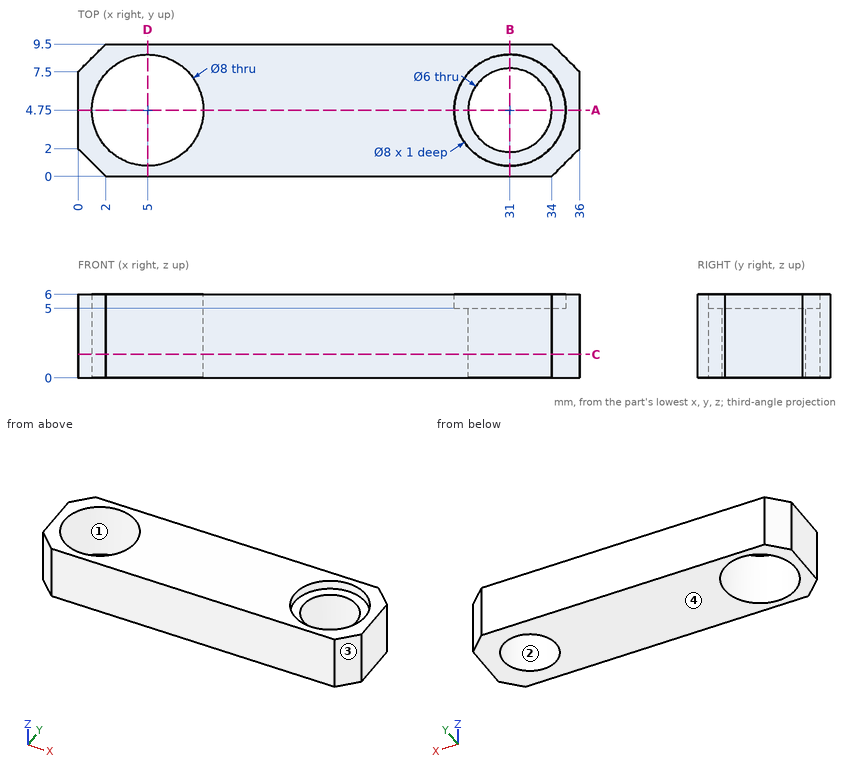
The drawing under review shows one solid part. Ordinate dimensions are in mm from its lowest x, y, z. Round coordinates to 2 decimals unless told otherwise and drop trailing zeros. Loops run counter-clockwise (first coordinate to the right, second up) from the corner with the lowest first, then second, coordinate; pieces in that order, holes last. Notation, with made-up numbers: (16.5, 41.25) - (50.5, 41.25) arc R26 ccw to (50.5, 71.25) - close; hole circle Ø9 at (38.25, 82). An arc over 180 degrees is marked (long way). Use a Markdown table: item, result. Add a question column.
Q1. For probe 1 along X at (y, z) = (4.25, 2.8); probe 2 along X at (y, z) = (7, 3.25); probe 3 along Y at (x, z) = (31, 5.2), list the stretches that pass through material, from the lowest coordinate up.
Q2. Add section C-C (z = 1.7). State the section outline as (x, y) points, plus the area to 3 significant figures.
Q3. The part is to be moulded in two halves that separate along X. For the marked faces 1, 2, 3 and 4, say which applies: pulls with the +X half, pulls with the -X half, needs draft (parallel to the pull), parting line crosses it, or undercut.
Q4. Add section D-D (x = 5). State the section outline as (y, z) points.
Q5. Add section B-B (x = 31). State the section outline as (y, z) points.
Q6. Add section A-A (y = 4.75). State the section outline as (x, z) points.
Worked answers:
| question | item | result |
|---|---|---|
| 1 | probe 1 | 0 to 1.03, 8.97 to 28.04, 33.96 to 36 |
| 1 | probe 2 | 0 to 1.69, 8.31 to 29.02, 32.98 to 36 |
| 1 | probe 3 | 0 to 0.75, 8.75 to 9.5 |
| 2 | outline | (0, 2) - (2, 0) - (34, 0) - (36, 2) - (36, 7.5) - (34, 9.5) - (2, 9.5) - (0, 7.5) - close; hole circle Ø8 at (5, 4.75); hole circle Ø6 at (31, 4.75) |
| 2 | area | 255 mm² |
| 3 | face 1 | undercut |
| 3 | face 2 | undercut |
| 3 | face 3 | pulls with the +X half |
| 3 | face 4 | needs draft |
| 4 | outline | (0, 0) - (0.75, 0) - (0.75, 6) - (0, 6) - close; (8.75, 0) - (9.5, 0) - (9.5, 6) - (8.75, 6) - close |
| 5 | outline | (0, 0) - (1.75, 0) - (1.75, 5) - (0.75, 5) - (0.75, 6) - (0, 6) - close; (7.75, 0) - (9.5, 0) - (9.5, 6) - (8.75, 6) - (8.75, 5) - (7.75, 5) - close |
| 6 | outline | (0, 0) - (1, 0) - (1, 6) - (0, 6) - close; (9, 0) - (28, 0) - (28, 5) - (27, 5) - (27, 6) - (9, 6) - close; (34, 0) - (36, 0) - (36, 6) - (35, 6) - (35, 5) - (34, 5) - close |
